```python
from build123d import *

# Parameters (mm, degrees)
SKETCH_1_W      = 78
SKETCH_1_H      = 20
EXTRUDE_1_DEPTH = 21.5
SHELL_1_T       = -2


with BuildPart() as part:
    # Эскиз1 → Бобышка-Вытянуть1 (new body)
    with BuildSketch(Plane(origin=(0, 0, 0), x_dir=(1, 0, 0), z_dir=(0, 1, 0))):
        Rectangle(SKETCH_1_W, SKETCH_1_H)
    extrude(amount=EXTRUDE_1_DEPTH)

    # Оболочка1
    shell_1_openings = [part.faces().sort_by_distance(p)[0] for p in [
        (0, 21.5, 0),
    ]]
    offset(amount=SHELL_1_T, openings=shell_1_openings, kind=Kind.INTERSECTION)


solid = part.part
```
CAD build for the part. Positions are in the model's coordinates, mm. A direction names the side the tool comes from. Give positions to 0.01 mm unless a question says otherwise; leave off trailing zeros. Write each loop counter-clockwise with the first axis right and the second up, starting at its lowest first coordinate (ties: lowest second). Pieces come first, ordered by that corner, then holes. Notation, with made-up numbers: (6, -13) -> (52, -13) arc R23 cw to (52, 0) -> close; hole circle Ø1 at (78, 9.25). An arc over 180 degrees is marked (long way). Write each question's results on one line, items separated by ' | '.
1. Cut at A-A, the plane y = 5.5. Write the cut outline in (x, z).
Geometry check:
outline: (-39, -10) -> (39, -10) -> (39, 10) -> (-39, 10) -> close; hole (-37, -8) -> (37, -8) -> (37, 8) -> (-37, 8) -> close
2. Cut at C-C, the plane x = 3. Write the cut outline in (y, z).
Geometry check:
outline: (0, -10) -> (21.5, -10) -> (21.5, -8) -> (2, -8) -> (2, 8) -> (21.5, 8) -> (21.5, 10) -> (0, 10) -> close
3. Cut at B-B, the plane z = -1.5. Write the cut outline in (x, y).
Geometry check:
outline: (-39, 0) -> (39, 0) -> (39, 21.5) -> (37, 21.5) -> (37, 2) -> (-37, 2) -> (-37, 21.5) -> (-39, 21.5) -> close
4. Drop a flat-ended pin along its axis: P1, Ø8, axis at x = -1.5, z = -0.5, coming from the +Y side. Give the stop position or say it passes through.
Geometry check:
P1: y = 2
5. Two-plate mould, pull along Z, no slides. Class faces 1 (the flat face through (-39, 11, 0)), 2 (the flat face through (-37, 12, 0)), 3 (the flat face through (-1, 11, 10)), 4 (the flat face through (-1, 12, -8)): pulls with the +Z half, pulls with the -Z half, needs draft (parallel to the pull), parting line crosses it, or undercut.
Geometry check:
face 1: needs draft | face 2: undercut | face 3: pulls with the +Z half | face 4: undercut
6. Wall check: probe 1 along X at (y, z) = (15, -7.75); probe 2 along Z at (x, y) = (-5, 3.5); probe 3 along Y at (x, z) = (-24.5, -4.25). Give the ranges that are in metal, low to high. Write a range as [from, to].
Geometry check:
probe 1: [-39, -37], [37, 39] | probe 2: [-10, -8], [8, 10] | probe 3: [0, 2]
7. Which spindle directions (+Z, -Z, +X, -X, +Y, -Y) get a long thin tool onto all of the face, cutting with end or side? Do faces 5 (the flat face through (-1, 11, -10)), 6 (the flat face through (-1, 12, 8)). Say none if no direction does.
Geometry check:
face 5: -Z, +X, -X, +Y, -Y | face 6: +Y
